from build123d import *

# Parameters (mm, degrees)
ESQUISSE1_W             = 35.6
ESQUISSE1_H             = 9.9
BOSS_EXTRU_1_DEPTH      = 3.9
ESQUISSE2_W             = 2.7
ESQUISSE2_H             = 1.5
ENL_V_MAT_EXTRU_1_DEPTH = 36.6
ESQUISSE3_W             = 35.6
ESQUISSE3_H             = 0.6
BOSS_EXTRU_2_DEPTH      = 1
CONG_1_R                = 0.2


with BuildPart() as part:
    # Esquisse1 → Boss.-Extru.1 (new body)
    with BuildSketch(Plane(origin=(0, 0, 0), x_dir=(1, 0, 0), z_dir=(0, 1, 0))):
        with Locations((17.8, 4.95)):
            Rectangle(ESQUISSE1_W, ESQUISSE1_H)
    extrude(amount=BOSS_EXTRU_1_DEPTH)

    # Esquisse2 → Enlèv. mat.-Extru.1 (cut, through all)
    with BuildSketch(Plane(origin=(35.6, 0, 0), x_dir=(0, 0, -1), z_dir=(1, 0, 0))):
        with Locations((4.95, 0.75)):
            Rectangle(ESQUISSE2_W, ESQUISSE2_H)
    extrude(amount=-ENL_V_MAT_EXTRU_1_DEPTH, mode=Mode.SUBTRACT)

    # Esquisse3 → Boss.-Extru.2 (add)
    with BuildSketch(Plane(origin=(0, 3.9, 0), x_dir=(1, 0, 0), z_dir=(0, 1, 0))):
        with Locations((17.8, 0.3)):
            Rectangle(ESQUISSE3_W, ESQUISSE3_H)
        with Locations((17.8, 9.6)):
            Rectangle(ESQUISSE3_W, ESQUISSE3_H)
    extrude(amount=BOSS_EXTRU_2_DEPTH)

    # Congé1
    cong_1_edges = [part.edges().sort_by_distance(p)[0] for p in [
        (0, 2.45, -9.9),
        (35.6, 2.45, -9.9),
        (35.6, 2.45, 0),
        (0, 2.45, 0),
    ]]
    fillet(cong_1_edges, radius=CONG_1_R)


solid = part.part
Could you check a few things on this model? Use its own coordinates, in mm. A direction names the side the tool comes from. Give positions to 0.01 mm unless a question says otherwise; leave off trailing zeros. Order: outer loops, then holes, each group sorted by start corner. A loop starts at its lowest first (then second) coordinate and runs counter-clockwise, first axis right, second up. Notation, with made-up numbers: (87, 35) -> (142, 35) arc R7 ccw to (142, 40) -> close; hole circle Ø7 at (23.25, 87). An arc over 180 degrees is marked (long way). Answer in a Markdown table with one row per item. Add a question column.
Item 1: Imagine slicing it at D-D (z = -7.75). List the corners of the cut face in (x, y) for me.
Item 2: Imagine slicing it at A-A (y = 0.7). List the corners of the cut face in (x, z) for me, and give its area (3 significant figures).
Item 3: Please list where these lines run through material, in increasing order: probe 1 along Z at (x, y) = (14.5, 0.5); probe 2 along Y at (x, z) = (28.5, -3.5); probe 3 along Z at (x, y) = (33, 4.6).
Item 4: We'd pull the mould along Z, two halves only. Please class faces 1 (the flat face through (18, 1.5, -5)), 2 (the flat face through (0, 2, -5)), 3 (the flat face through (18, 2, 0)): pulls with the +Z half, pulls with the -Z half, needs draft (parallel to the pull), parting line crosses it, or undercut.
Item 5: For faces 4 (the flat face through (17.6, 4.4, -0.6)), 5 (the flat face through (18, 1, -6.3)), 6 (the flat face through (18, 0, -2)), which set-ups out of +Z, -Z, +X, -X, +Y, -Y let a thin tool reach every point of the face, with its end or its side?
Item 6: I'm going to push flat-ended pins straight in: P1, Ø2.5, axis at x = 22, z = -4.5, coming from the +Y side; P2, Ø2, axis at x = 13, z = -5, coming from the -Y side. Where does each tip first touch, or does it pass through?
Item 7: Imagine slicing it at C-C (z = -4). List the corners of the cut face in (x, y) for me, and give its area (3 significant figures).
Item 8: Imagine slicing it at B-B (x = 13). List the corners of the cut face in (y, z) for me, and give its area (3 significant figures).
Result:
| question | item | result |
|---|---|---|
| 1 | outline | (0, 0) -> (35.6, 0) -> (35.6, 3.9) -> (0, 3.9) -> close |
| 2 | outline | (0, -9.7) arc R0.2 ccw to (0.2, -9.9) -> (35.4, -9.9) arc R0.2 ccw to (35.6, -9.7) -> (35.6, -6.3) -> (0, -6.3) -> close; (0, -3.6) -> (35.6, -3.6) -> (35.6, -0.2) arc R0.2 ccw to (35.4, 0) -> (0.2, 0) arc R0.2 ccw to (0, -0.2) -> close |
| 2 | area | 256 mm2 |
| 3 | probe 1 | -9.9 to -6.3, -3.6 to 0 |
| 3 | probe 2 | 0 to 3.9 |
| 3 | probe 3 | -9.9 to -9.3, -0.6 to 0 |
| 4 | face 1 | undercut |
| 4 | face 2 | needs draft |
| 4 | face 3 | pulls with the +Z half |
| 5 | face 4 | +X, -X, +Y |
| 5 | face 5 | +X, -X, -Y |
| 5 | face 6 | +Z, -Z, +X, -X, -Y |
| 6 | P1 | y = 3.9 |
| 6 | P2 | y = 1.5 |
| 7 | outline | (0, 1.5) -> (35.6, 1.5) -> (35.6, 3.9) -> (0, 3.9) -> close |
| 7 | area | 85.4 mm2 |
| 8 | outline | (0, -9.9) -> (4.9, -9.9) -> (4.9, -9.3) -> (3.9, -9.3) -> (3.9, -0.6) -> (4.9, -0.6) -> (4.9, 0) -> (0, 0) -> (0, -3.6) -> (1.5, -3.6) -> (1.5, -6.3) -> (0, -6.3) -> close |
| 8 | area | 35.8 mm2 |
